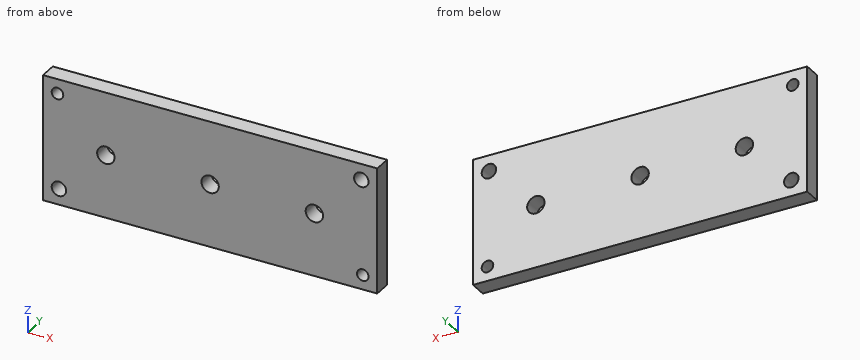
```python
from build123d import *

# Parameters (mm, degrees)
SKETCH1_W           = 57.7
SKETCH1_H           = 21.7
BOSS_EXTRUDE1_DEPTH = 2
SKETCH2_W           = 57.7
SKETCH2_H           = 21.7
SKETCH2_W_2         = 54.7
SKETCH2_H_2         = 18.7
BOSS_EXTRUDE2_DEPTH = 75
FILLET1_R           = 8
SKETCH3_W           = 38.583587397
SKETCH3_H           = 2.5
CUT_EXTRUDE1_DEPTH  = 75
SKETCH4_W           = 17.089400488
SKETCH4_H           = 2.5
CUT_EXTRUDE2_DEPTH  = 75
SKETCH5_R           = 1
CUT_EXTRUDE3_DEPTH  = 8
BOSS_EXTRUDE3_START = 3
SKETCH6_W           = 57.7
SKETCH6_H           = 21.7
SKETCH6_R           = 1
SKETCH6_R_2         = 1.25
BOSS_EXTRUDE3_DEPTH = 3
CUT_EXTRUDE4_DEPTH  = 3
CUT_EXTRUDE5_START  = -3
SKETCH8_R           = 1.5
CUT_EXTRUDE5_DEPTH  = 3
SKETCH9_W           = 91.990762183
SKETCH9_H           = 98.377858587
CUT_EXTRUDE7_DEPTH  = 69


with BuildPart() as part:
    # Sketch1 → Boss-Extrude1 (new body)
    with BuildSketch(Plane(origin=(0, 0, 0), x_dir=(1, 0, 0), z_dir=(0, 1, 0))):
        with Locations((28.85, 10.85)):
            Rectangle(SKETCH1_W, SKETCH1_H)
    extrude(amount=BOSS_EXTRUDE1_DEPTH)

    # Sketch2 → Boss-Extrude2 (add)
    with BuildSketch(Plane(origin=(0, 2, 0), x_dir=(1, 0, 0), z_dir=(0, 1, 0))):
        with Locations((28.85, 10.85)):
            Rectangle(SKETCH2_W, SKETCH2_H)
        with Locations((28.85, 10.85)):
            Rectangle(SKETCH2_W_2, SKETCH2_H_2, mode=Mode.SUBTRACT)
    extrude(amount=BOSS_EXTRUDE2_DEPTH)

    # Fillet1
    fillet1_edges = [part.edges().sort_by_distance(p)[0] for p in [
        (1.5, 39.5, -20.2),
        (1.5, 39.5, -1.5),
        (56.2, 39.5, -1.5),
        (56.2, 39.5, -20.2),
    ]]
    fillet(fillet1_edges, radius=FILLET1_R)

    # Sketch3 → Cut-Extrude1 (cut)
    with BuildSketch(Plane(origin=(0, 77, 0), x_dir=(1, 0, 0), z_dir=(0, 1, 0))):
        with Locations((20.791793699, 18.95)):
            Rectangle(SKETCH3_W, SKETCH3_H)
    extrude(amount=-CUT_EXTRUDE1_DEPTH, mode=Mode.SUBTRACT)

    # Sketch4 → Cut-Extrude2 (cut)
    with BuildSketch(Plane(origin=(0, 77, 0), x_dir=(1, 0, 0), z_dir=(0, 1, 0))):
        with Locations((47.655299756, 2.75)):
            Rectangle(SKETCH4_W, SKETCH4_H)
    extrude(amount=-CUT_EXTRUDE2_DEPTH, mode=Mode.SUBTRACT)

    # Sketch5 → Cut-Extrude3 (cut)
    with BuildSketch(Plane(origin=(0, 77, 0), x_dir=(1, 0, 0), z_dir=(0, 1, 0))):
        with Locations(Location((55.2, 19.2, 0), (0, 0, 270))):
            Circle(SKETCH5_R)
        with Locations(Location((2.5, 2.5, 0), (0, 0, 270))):
            Circle(SKETCH5_R)
    extrude(amount=-CUT_EXTRUDE3_DEPTH, mode=Mode.SUBTRACT)

    # Sketch6 → Boss-Extrude3 (add)
    with BuildSketch(Plane(origin=(0, 77, 0), x_dir=(1, 0, 0), z_dir=(0, 1, 0)).offset(BOSS_EXTRUDE3_START)):
        with Locations((28.85, 10.85)):
            Rectangle(SKETCH6_W, SKETCH6_H)
        with Locations(Location((2.5, 2.5, 0), (0, 0, 270))):
            Circle(SKETCH6_R, mode=Mode.SUBTRACT)
        with Locations(Location((55.2, 19.2, 0), (0, 0, 270))):
            Circle(SKETCH6_R, mode=Mode.SUBTRACT)
        with Locations(Location((2.75, 18.95, 0), (0, 0, 270))):
            Circle(SKETCH6_R_2, mode=Mode.SUBTRACT)
        with Locations(Location((54.95, 2.75, 0), (0, 0, 270))):
            Circle(SKETCH6_R_2, mode=Mode.SUBTRACT)
    extrude(amount=-BOSS_EXTRUDE3_DEPTH)

    # Sketch7 → Cut-Extrude4 (cut)
    with BuildSketch(Plane(origin=(0, 80, 0), x_dir=(1, 0, 0), z_dir=(0, 1, 0))):
        with BuildLine():
            ThreePointArc((9.35, 10.85), (10.85, 9.35), (12.35, 10.85))
            Line((12.35, 10.85), (10.85, 10.85))
            Line((10.85, 10.85), (9.35, 10.85))
        make_face()
        with BuildLine():
            Line((10.85, 10.85), (12.35, 10.85))
            ThreePointArc((12.35, 10.85), (10.85, 12.35), (9.35, 10.85))
            Line((9.35, 10.85), (10.85, 10.85))
        make_face()
        with BuildLine():
            ThreePointArc((27.35, 10.85), (28.85, 9.35), (30.35, 10.85))
            Line((30.35, 10.85), (28.85, 10.85))
            Line((28.85, 10.85), (27.35, 10.85))
        make_face()
        with BuildLine():
            Line((28.85, 10.85), (30.35, 10.85))
            ThreePointArc((30.35, 10.85), (28.85, 12.35), (27.35, 10.85))
            Line((27.35, 10.85), (28.85, 10.85))
        make_face()
        with BuildLine():
            ThreePointArc((45.35, 10.85), (46.85, 9.35), (48.35, 10.85))
            Line((48.35, 10.85), (46.85, 10.85))
            Line((46.85, 10.85), (45.35, 10.85))
        make_face()
        with BuildLine():
            Line((46.85, 10.85), (48.35, 10.85))
            ThreePointArc((48.35, 10.85), (46.85, 12.35), (45.35, 10.85))
            Line((45.35, 10.85), (46.85, 10.85))
        make_face()
    extrude(amount=-CUT_EXTRUDE4_DEPTH, mode=Mode.SUBTRACT)

    # Sketch8 → Cut-Extrude5 (cut)
    with BuildSketch(Plane.XZ.offset(CUT_EXTRUDE5_START)):
        with Locations(Location((10.85, -10.85, 0), (0, 0, 90))):
            Circle(SKETCH8_R)
        with Locations(Location((28.85, -10.85, 0), (0, 0, 90))):
            Circle(SKETCH8_R)
        with Locations(Location((46.85, -10.85, 0), (0, 0, 90))):
            Circle(SKETCH8_R)
    extrude(amount=CUT_EXTRUDE5_DEPTH, mode=Mode.SUBTRACT)

    # Sketch9 → Cut-Extrude7 (cut)
    with BuildSketch(Plane(origin=(0, 0, -21.7), x_dir=(-1, 0, 0), z_dir=(0, 0, -1))):
        with Locations((-24.534497704, 27.811070706)):
            Rectangle(SKETCH9_W, SKETCH9_H)
    extrude(amount=-CUT_EXTRUDE7_DEPTH, mode=Mode.SUBTRACT)


solid = part.part
```
Source: CAD feature listing. Evaluate the final solid. Frame: model axes, mm. Coordinates: 2 decimals unless noted, no trailing zeros. Order: outer loops, then holes, each group sorted by start corner. A loop starts at its lowest first (then second) coordinate and runs counter-clockwise, first axis right, second up. Notation, with made-up numbers: (-37, 8.5) - (5, 8.5) arc R31 ccw to (5, 32.5) - close; hole circle Ø2 at (78, 83.25). An arc over 180 degrees is marked (long way). One line per item, written item: value.
1) Cut plane A-A on x = 28.85. Output: boundary loops of the cut face in (y, z).
Computed values:
outline: (77, -21.7) - (80, -21.7) - (80, -12.35) - (77, -12.35) - close; (77, -9.35) - (80, -9.35) - (80, 0) - (77, 0) - close
2) Ray query, line 1 (X direction, y = 78.95, z = -10.85); line 2 (X direction, y = 78.5, z = -2.75); line 3 (Z direction, x = 10.85, y = 78.5). Return the intervals inside material, ascending. Write a range as [from, to].
Computed values:
line 1: x = [0, 9.35], [12.35, 27.35], [30.35, 45.35], [48.35, 57.7]
line 2: x = [0, 1.53], [3.47, 53.7], [56.2, 57.7]
line 3: z = [-21.7, -12.35], [-9.35, 0]
3) Cut plane B-B on y = 79.4. Output: boundary loops of the cut face in (x, z).
Computed values:
outline: (0, -21.7) - (57.7, -21.7) - (57.7, 0) - (0, 0) - close; hole circle Ø2.5 at (2.75, -18.95); hole circle Ø2 at (2.5, -2.5); hole circle Ø3 at (10.85, -10.85); hole circle Ø3 at (28.85, -10.85); hole circle Ø3 at (46.85, -10.85); hole circle Ø2.5 at (54.95, -2.75); hole circle Ø2 at (55.2, -19.2)
4) Cut plane C-C on z = -2.75. Output: boundary loops of the cut face in (x, y), plus the area to 3 significant figures.
Computed values:
outline: (0, 77) - (1.53, 77) - (1.53, 80) - (0, 80) - close; (3.47, 77) - (53.7, 77) - (53.7, 80) - (3.47, 80) - close; (56.2, 77) - (57.7, 77) - (57.7, 80) - (56.2, 80) - close
area: 160 mm^2
5) Contact query for a flat-ended pin moving along its axis: pin 1 (2 mm diameter, centred on x = 2.75, z = -18.95, fed in from -Y). Output: stop coordinate, or through.
Computed values:
pin 1: passes through
